```python
from build123d import *

# Parameters (mm, degrees)
F2_R     = 0.9
F3_DEPTH = 2.5
F4_R     = 3
F5_DEPTH = 2.5
F6_R     = 1.75
F7_DEPTH = 10.0710001


with BuildPart() as f1:
    # F0 (on Front) → F1 (revolve)
    with BuildSketch(Plane.XZ):
        Polygon((14, -35.9), (23.5, -35.9), (23.5, -33.9), (27.5, -33.9), (27.5, -30.8), (25.75, -30.8), (25.75, -27.8), (23.9, -27.8), (23.9, -26.8), (22.6261041801, -26.8), (23.9, -23.3), (23.9, -22.8), (19, -22.8), (14, -33.4), align=None)
    revolve(axis=Axis((0, 0, -3.8875962891), (0, 0, -1)))

    # F2 (on face) → F3 (cut)
    with BuildSketch(Plane(origin=(0, 0, -35.9), x_dir=(1, 0, 0), z_dir=(0, 0, -1))):
        with Locations((3.2437529214, 16.6876621186)):
            Circle(F2_R)
        with Locations((16.0738157852, -5.5346586258)):
            Circle(F2_R)
        with Locations((-16.0738157852, -5.5346586258)):
            Circle(F2_R)
    extrude(amount=-F3_DEPTH, mode=Mode.SUBTRACT)

    # F4 (on face) → F5 (cut)
    with BuildSketch(Plane(origin=(0, 0, -35.9), x_dir=(1, 0, 0), z_dir=(0, 0, -1))):
        with BuildLine():
            Line((22, -2.0093531297), (22, 2.0093531297))
            ThreePointArc((22, 2.0093531297), (17.75, 0), (22, -2.0093531297))
        make_face()
        with Locations((-3.6643229153, 17.6230740103)):
            Circle(F4_R)
        with Locations((0, -16.5)):
            Circle(F4_R)
    extrude(amount=-F5_DEPTH, mode=Mode.SUBTRACT)

    # F6 (on face) → F7 (cut, through all)
    with BuildSketch(Plane(origin=(0, 0, -33.4), x_dir=(1, 0, 0), z_dir=(0, 0, -1))):
        with Locations((3.2437529214, 16.6876621186)):
            Circle(F6_R)
        with Locations((-16.0738157852, -5.5346586258)):
            Circle(F6_R)
        with Locations((16.0738157852, -5.5346586258)):
            Circle(F6_R)
    extrude(amount=-F7_DEPTH, mode=Mode.SUBTRACT)


solid = f1.part
```
Build history of the part. All positions in model axes, mm. A direction names the side the tool comes from. Round coordinates to 2 decimals unless told otherwise and drop trailing zeros. Write each loop counter-clockwise with the first axis right and the second up, starting at its lowest first coordinate (ties: lowest second). Pieces come first, ordered by that corner, then holes.
1) Mould opens along Y. For faces 1 (the cylindrical face through (12.85, -20.15, -27.29)), 2 (the flat face through (2, -17, -33.4)), 3 (the flat face through (8, 23, -27.8)) say: +Y half, -Y half, draft (parallel to the pull), parting line (faces both ways), or undercut.
2) 3-axis set-ups, long thin cutter, end or side, ignore diameter. For faces 4 (the cylindrical face through (-6.66, -17.75, -34.67)), 5 (the flat face through (-14, 18, -26.8)), 6 (the flat face through (15, 5, -33.4)): which of +Z, -Z, +X, -X, +Y, -Y reach the whole face in a straight line?
3) Drill centre lines: probe 1 along X at (y, z) = (0, -34.2); probe 2 along Z at (x, y) = (-11, 21.5); probe 3 along Y at (x, z) = (-15, -31.75). Where is each one in solid material? Low to high.
4) Band-saw the part on B-B, the plane z = -25.25. List the corners of the cut face in (x, y), and give its area (3 significant figures).
5) Pin check, flat tips, straight feed: pin 1 (1.5 mm diameter, centred on y = 11, z = -33, fed in from +X); pin 2 (9.5 mm diameter, centred on x = 0, y = 16.5, fed in from +Z); pin 3 (4 mm diameter, centred on y = -2.5, z = -27.5, fed in from +X); pin 4 (4 mm diameter, centred on x = 17, z = -24, fed in from +Y). Stop position of each tip, or through.
Ans:
1. face 1: parting line
1. face 2: undercut
1. face 3: draft
2. face 4: -Z
2. face 5: none
2. face 6: +Z
3. probe 1: x = -23.5 to -14, 14 to 17.75, 22 to 23.5
3. probe 2: z = -33.9 to -27.8
3. probe 3: y = -23.05 to 4.15, 6.92 to 23.05
4. outline: circle Ø46.38 at (0, 0); hole (-17.32, 4.3) arc R17.84 ccw to (1.85, -17.75) arc R1.75 ccw to (4.93, -17.15) arc R17.84 ccw to (17.32, 4.3) arc R1.75 ccw to (16.3, 7.27) arc R17.84 ccw to (-16.3, 7.27) arc R1.75 ccw to start
4. area: 683 mm2
5. pin 1: stops at x = 25.52
5. pin 2: stops at z = -22.8
5. pin 3: stops at x = 25.74
5. pin 4: stops at y = 18.5
